Can you work these out from the model? Positions are in its coordinate system, mm. Round coordinates to 2 decimals unless told otherwise and drop trailing zeros. Loops run counter-clockwise (first coordinate to the right, second up) from the corner with the lowest first, then second, coordinate; pieces in that order, holes last. Notation, with made-up numbers: M 50.25,-19 L 90.25,-19 A23 cw 90.25,2 Z; hole C -3,60.5 d11. An arc over 180 degrees is marked long. Return JSON: item names as keys, results as strings.
```python
from build123d import *

# Parameters (mm, degrees)
PAD_DEPTH = 3


with BuildPart() as part:
    # Sketch → Pad (new body)
    with BuildSketch(Plane.XZ):
        Polygon((-29.947879, 9.404758), (39.852381, 9.404758), (39.852381, 20.041461), (59.928709, 0), (40.015407, -20.117136), (40.015407, -10.023776), (-29.947879, -10.023776), align=None)
    extrude(amount=PAD_DEPTH)


solid = part.part
```
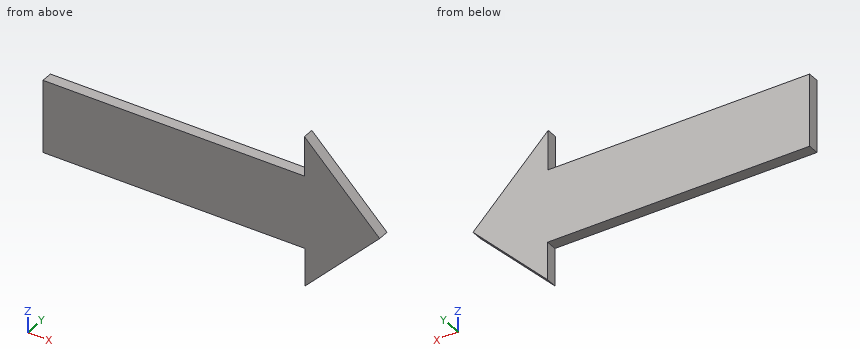
Q1. Suppose I cut it at A-A, the plane y = -1.9. Please give me the cut outline in (x, z).
Results:
{"outline": "M -29.95,-10.02 L 40.02,-10.02 L 40.02,-20.12 L 59.93,0 L 39.85,20.04 L 39.85,9.4 L -29.95,9.4 Z"}
Q2. I'm going to push flat-ended pins straight in: pin 1 Ø1.5 at (x, y) = (16.5, -2) entering from +Z; pin 2 Ø2 at (x, z) = (-9, 10.5) entering from +Y; pin 3 Ø0.9 at (y, z) = (-1, 14) entering from -X; pin 4 Ø1.5 at (x, y) = (-11, -0.5) entering from -Z. Where does each tip first touch, or does it pass through?
Results:
{"pin 1": "stops at z = 9.4", "pin 2": "passes through", "pin 3": "stops at x = 39.85", "pin 4": "stops at z = -10.02"}
Q3. Suppose I cut it at B-B, the plane x = 21.5. Please give me the cut outline in (y, z).
Results:
{"outline": "M -3,-10.02 L 0,-10.02 L 0,9.4 L -3,9.4 Z"}
Q4. If I drill on line 1 along Z through (x, y) = (-24, -2.75); line 2 along X through (y, z) = (-1.9, 7); line 3 along X through (y, z) = (-1.2, 12), over which ranges is the centre line in solid material (lowest first)?
Results:
{"line 1": "z = -10.02 to 9.4", "line 2": "x = -29.95 to 52.92", "line 3": "x = 39.85 to 47.91"}
Q5. Suppose I cut it at C-C, the plane z = 3. Please give me the cut outline in (x, y), plus the area to 3 significant figures.
Results:
{"outline": "M -29.95,-3 L 56.92,-3 L 56.92,0 L -29.95,0 Z", "area": "261 mm2"}
